from build123d import *

# Parameters (mm, degrees)
FILLET1_R   = 0.2
HEX_START   = -2.3
HEX_2_DEPTH = 2.3


with BuildPart() as part:
    # BodySke → BaseBody (revolve)
    with BuildSketch(Plane.XY, mode=Mode.PRIVATE) as basebody_sk:
        Polygon((0, 0), (0, 4.82), (0.48, 4.82), (2.8, 2.5), (11.555, 2.5), (12, 2.055), (12, 0), align=None)
    revolve(basebody_sk.sketch.rotate(Axis((0, 0, 0), (1, 0, 0)), 90), axis=Axis((0, 0, 0), (1, 0, 0)))

    # Fillet1
    fillet1_edges = [part.edges().sort_by_distance(p)[0] for p in [
        (2.8, 0, -2.5),
    ]]
    fillet(fillet1_edges, radius=FILLET1_R)

    # Hex 2: read off the stored shape, not the designer's step
    # Hex 2 outline → Hex 2 (cut)
    with BuildSketch(Plane.ZY.offset(HEX_START)):
        Polygon((-1.51, -0.871798906), (0, -1.743597813), (1.51, -0.871798906), (1.51, 0.871798906), (0, 1.743597813), (-1.51, 0.871798906), align=None)
    extrude(amount=HEX_2_DEPTH, mode=Mode.SUBTRACT)

    # Hex 2 2 outline → Hex 2 2 (revolve, cut)
    with BuildSketch(Plane.YX):
        Polygon((1.51, 2.3), (0, 3.171798906), (0, 2.3), align=None)
    revolve(axis=Axis((0, 0, 0), (1, 0, 0)), mode=Mode.SUBTRACT)


solid = part.part
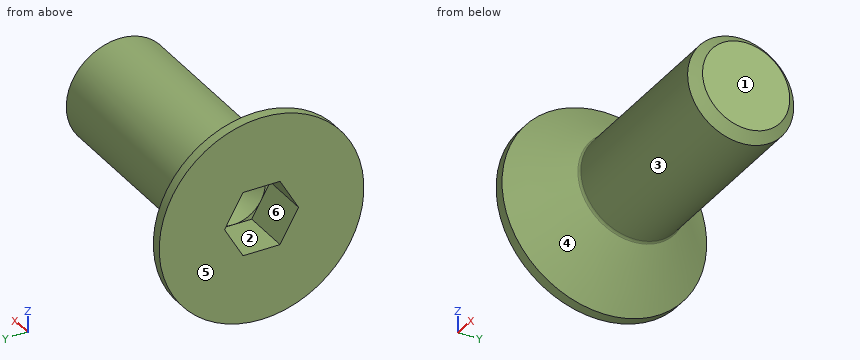
Design review of the part built by this model. Coordinates are the model's own, in mm. Face numbers are marked on the shaded views. A direction names the side the tool comes from. Round coordinates to 2 decimals unless told otherwise and drop trailing zeros. Write each loop counter-clockwise with the first axis right and the second up, starting at its lowest first coordinate (ties: lowest second). Pieces come first, ordered by that corner, then holes. Notation, with made-up numbers: (-15.5, 1) - (2.5, 1) arc R17 cw to (2.5, 11) - close; hole circle Ø8 at (41.5, 76.5). An arc over 180 degrees is marked (long way). Use a Markdown table: item, result. Add a question column.
1. For the marked faces 1, 2 and 3, list the 3-axis set-ups (+Z, -Z, +X, -X, +Y, -Y) from which the entire face can be reached by the end or side of a thin tool; tool diameter is ignored.
2. Wall thickness on probe 1 along Y at (x, z) = (10.25, 0); probe 2 along Z at (x, y) = (10.75, -0.5); probe 3 along Y at (x, z) = (11.5, -1.25): over which ranges is each line inside the solid? List them lowest first.
3. Mouldability with a two-part tool opening along Y and no side actions: class the marked faces 4, 5 and 6 as +Y half, -Y half, draft (parallel to the pull), parting line (faces both ways), or undercut.
4. We need section B-B (x = 2.5). State the section outline as (y, z) points, then the cut area to 3 significant figures.
5. Clearance check with flat-ended pins moving along their axes: pin 1 (3 mm diameter, centred on x = 8.5, y = -3, fed in from -Z); pin 2 (3 mm diameter, centred on x = 3.5, y = 3, fed in from -Z); pin 3 (5 mm diameter, centred on x = 3, y = 3.5, fed in from +Z). State where each tip first meets the part, or that it passes through.
6. We need section A-A (x = 8). State the section outline as (y, z) points.
Output:
| question | item | result |
|---|---|---|
| 1 | face 1 | +Z, -Z, +X, +Y, -Y |
| 1 | face 2 | -X |
| 1 | face 3 | +X |
| 2 | probe 1 | y = -2.5 to 2.5 |
| 2 | probe 2 | z = -2.45 to 2.45 |
| 2 | probe 3 | y = -2.17 to 2.17 |
| 3 | face 4 | parting line |
| 3 | face 5 | draft |
| 3 | face 6 | undercut |
| 4 | outline | circle Ø5.6 at (0, 0); hole circle Ø2.33 at (0, 0) |
| 4 | area | 20.4 mm2 |
| 5 | pin 1 | stops at z = -2 |
| 5 | pin 2 | stops at z = -2.14 |
| 5 | pin 3 | stops at z = 3.86 |
| 6 | outline | circle Ø5 at (0, 0) |
